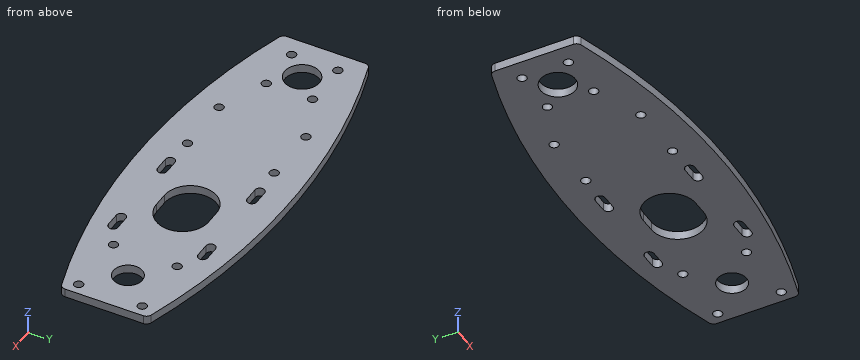
```python
from build123d import *

# Parameters (mm, degrees)
MODEL_R         = 5
MODEL_R_2       = 6
MODEL_R_3       = 1.575
EXTRUDE_1_DEPTH = 3


with BuildPart() as part:
    # Model → 凸台-拉伸1 (new body)
    with BuildSketch(Plane.XY):
        with BuildLine():
            Line((-88, 13.542891419), (-88, -13.542891419))
            ThreePointArc((-88, -13.542891419), (-87.614574011, -14.723209496), (-86.606849237, -15.448602311))
            ThreePointArc((-86.606849237, -15.448602311), (-18, -26.108381092), (50.606849237, -15.448602311))
            ThreePointArc((50.606849237, -15.448602311), (51.614574011, -14.723209496), (52, -13.542891419))
            Line((52, -13.542891419), (52, 13.542891419))
            ThreePointArc((52, 13.542891419), (51.614574011, 14.723209496), (50.606849237, 15.448602311))
            ThreePointArc((50.606849237, 15.448602311), (-18, 26.108381092), (-86.606849237, 15.448602311))
            ThreePointArc((-86.606849237, 15.448602311), (-87.614574011, 14.723209496), (-88, 13.542891419))
        make_face()
        with Locations((37, 0)):
            Circle(MODEL_R, mode=Mode.SUBTRACT)
        with Locations((-73, 0)):
            Circle(MODEL_R_2, mode=Mode.SUBTRACT)
        with Locations((26, 11)):
            Circle(MODEL_R_3, mode=Mode.SUBTRACT)
        with Locations((48, 11)):
            Circle(MODEL_R_3, mode=Mode.SUBTRACT)
        with Locations((48, -11)):
            Circle(MODEL_R_3, mode=Mode.SUBTRACT)
        with Locations((26, -11)):
            Circle(MODEL_R_3, mode=Mode.SUBTRACT)
        with Locations((-81, 8)):
            Circle(MODEL_R_3, mode=Mode.SUBTRACT)
        with Locations((-65, 8)):
            Circle(MODEL_R_3, mode=Mode.SUBTRACT)
        with Locations((-65, -8)):
            Circle(MODEL_R_3, mode=Mode.SUBTRACT)
        with Locations((-81, -8)):
            Circle(MODEL_R_3, mode=Mode.SUBTRACT)
        with Locations((-28, 15)):
            Circle(MODEL_R_3, mode=Mode.SUBTRACT)
        with Locations((-28, -15)):
            Circle(MODEL_R_3, mode=Mode.SUBTRACT)
        with Locations((-48, -15)):
            Circle(MODEL_R_3, mode=Mode.SUBTRACT)
        with Locations((-48, 15)):
            Circle(MODEL_R_3, mode=Mode.SUBTRACT)
        with BuildLine():
            Line((2.5, 9), (-2.5, 9))
            ThreePointArc((-2.5, 9), (-11.5, 0), (-2.5, -9))
            Line((-2.5, -9), (2.5, -9))
            ThreePointArc((2.5, -9), (11.5, 0), (2.5, 9))
        make_face(mode=Mode.SUBTRACT)
        with BuildLine():
            Line((-13, 17.15), (-18, 17.15))
            ThreePointArc((-18, 17.15), (-19.65, 15.5), (-18, 13.85))
            Line((-18, 13.85), (-13, 13.85))
            ThreePointArc((-13, 13.85), (-11.35, 15.5), (-13, 17.15))
        make_face(mode=Mode.SUBTRACT)
        with BuildLine():
            Line((18, 17.15), (13, 17.15))
            ThreePointArc((13, 17.15), (11.35, 15.5), (13, 13.85))
            Line((13, 13.85), (18, 13.85))
            ThreePointArc((18, 13.85), (19.65, 15.5), (18, 17.15))
        make_face(mode=Mode.SUBTRACT)
        with BuildLine():
            Line((13, -17.15), (18, -17.15))
            ThreePointArc((18, -17.15), (19.65, -15.5), (18, -13.85))
            Line((18, -13.85), (13, -13.85))
            ThreePointArc((13, -13.85), (11.35, -15.5), (13, -17.15))
        make_face(mode=Mode.SUBTRACT)
        with BuildLine():
            Line((-13, -13.85), (-18, -13.85))
            ThreePointArc((-18, -13.85), (-19.65, -15.5), (-18, -17.15))
            Line((-18, -17.15), (-13, -17.15))
            ThreePointArc((-13, -17.15), (-11.35, -15.5), (-13, -13.85))
        make_face(mode=Mode.SUBTRACT)
    extrude(amount=EXTRUDE_1_DEPTH)


solid = part.part
```
Geometry: final body of the model. Coordinates: model frame, mm. Round coordinates to 2 decimals unless told otherwise and drop trailing zeros. Loops run counter-clockwise (first coordinate to the right, second up) from the corner with the lowest first, then second, coordinate; pieces in that order, holes last. Notation, with made-up numbers: (-28.5, 46) -> (17.5, 46) arc R19 cw to (17.5, 56) -> close; hole circle Ø11 at (-33, 17). An arc over 180 degrees is marked (long way). Use one line per item in the form item = value.
Item 1: Material intervals for probe 1 along X at (y, z) = (7, 1.5); probe 2 along Y at (x, z) = (26, 1.55) (3 decimals); probe 3 along Y at (x, z) = (-47, 1.85), sorted ascending.
Evaluation:
probe_1 = -88 to -82.22, -79.78 to -66.22, -63.78 to -8.16, 8.16 to 52
probe_2 = -21.786 to -12.575, -9.425 to 9.425, 12.575 to 21.786
probe_3 = -24.24 to -16.22, -13.78 to 13.78, 16.22 to 24.24
Item 2: Cut plane B-B on x = -48. Output: boundary loops of the cut face in (y, z) (3 decimals), then the cut area to 3 significant figures.
Evaluation:
outline = (-24.109, 0) -> (-16.575, 0) -> (-16.575, 3) -> (-24.109, 3) -> close; (-13.425, 0) -> (13.425, 0) -> (13.425, 3) -> (-13.425, 3) -> close; (16.575, 0) -> (24.109, 0) -> (24.109, 3) -> (16.575, 3) -> close
area = 126 mm2
Item 3: Contact query for flat-ended pins moving along their axis: pin 1 Ø0.9 at (x, z) = (-15, 2) entering from -Y; pin 2 Ø1.5 at (x, z) = (-0.5, 1) entering from +Y. Output: stop coordinate, or through.
Evaluation:
pin_1 = -26.09
pin_2 = 25.49
Item 4: Cut plane C-C on x = 35. Output: boundary loops of the cut face in (y, z).
Evaluation:
outline = (-19.81, 0) -> (-4.58, 0) -> (-4.58, 3) -> (-19.81, 3) -> close; (4.58, 0) -> (19.81, 0) -> (19.81, 3) -> (4.58, 3) -> close
Item 5: Cut plane A-A on y = 11. Output: boundary loops of the cut face in (x, z) (3 decimals).
Evaluation:
outline = (-88, 0) -> (24.425, 0) -> (24.425, 3) -> (-88, 3) -> close; (27.575, 0) -> (46.425, 0) -> (46.425, 3) -> (27.575, 3) -> close; (49.575, 0) -> (52, 0) -> (52, 3) -> (49.575, 3) -> close
Item 6: Cut plane D-D on z = 0.85. Give the number of separate pieces and of enclosed holes in the cut face, then the cut area to 3 significant figures.
Evaluation:
separate_pieces = 1
enclosed_holes = 19
area = 5,550 mm2
